The figure shows three views and two pictorial views of one solid part (mm, origin at its lowest corner). Answer the questions. A direction names the side the tool comes from. Round coordinates to 2 decimals unless told otherwise and drop trailing zeros. Order: outer loops, then holes, each group sorted by start corner. A loop starts at its lowest first (then second) coordinate and runs counter-clockwise, first axis right, second up. Notation, with made-up numbers: M -18,30.5 L 13,30.5 A13 ccw 13,39.5 Z; hole C -27.5,-35 d9. An arc over 180 degrees is marked long. Return JSON: item names as keys, results as strings.
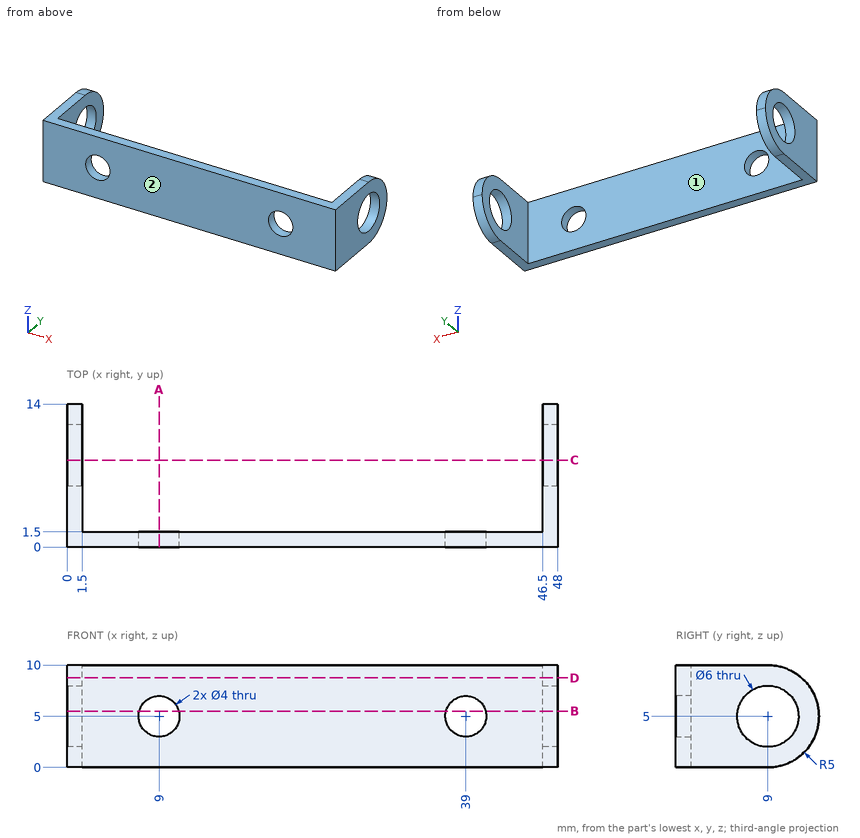
Item 1: Find section C-C (y = 8.5). Determine the outline of the cut face in (x, z).
Output:
{"outline": "M 0,0 L 1.5,0 L 1.5,2.04 L 0,2.04 Z; M 0,7.96 L 1.5,7.96 L 1.5,10 L 0,10 Z; M 46.5,0 L 48,0 L 48,2.04 L 46.5,2.04 Z; M 46.5,7.96 L 48,7.96 L 48,10 L 46.5,10 Z"}
Item 2: This flat-tipped pin is pushed along its axis until it touches: pin 1 (5 mm diameter, centred on x = 20, z = 3, fed in from +Y). Where does it stop, or does it pass through?
Output:
{"pin 1": "stops at y = 1.5"}
Item 3: Consider line 1 along X through (y, z) = (1, 5); line 2 along Y through (x, z) = (47.2, 5); line 3 along X through (y, z) = (3, 9). Determine where each line is inside the solid, lowest interval first. Write a range as [from, to].
Output:
{"line 1": "x = [0, 7], [11, 37], [41, 48]", "line 2": "y = [0, 6], [12, 14]", "line 3": "x = [0, 1.5], [46.5, 48]"}
Item 4: Which of the six approach directions +Z, -Z, +X, -X, +Y, -Y give full straight-line access (tool end or side, diameter ignored) to the marked faces 1 and 2?
Output:
{"face 1": "+Z, -Z, +Y", "face 2": "+Z, -Z, +X, -X, -Y"}
Item 5: Find section D-D (z = 8.75). Determine the outline of the cut face in (x, y), plus the area to 3 significant figures.
Output:
{"outline": "M 0,0 L 48,0 L 48,12.31 L 46.5,12.31 L 46.5,1.5 L 1.5,1.5 L 1.5,12.31 L 0,12.31 Z", "area": "104 mm^2"}
Item 6: Find section B-B (z = 5.5). Determine the outline of the cut face in (x, y), plus the area to 3 significant figures.
Output:
{"outline": "M 0,0 L 7.06,0 L 7.06,1.5 L 1.5,1.5 L 1.5,6.04 L 0,6.04 Z; M 0,11.96 L 1.5,11.96 L 1.5,13.97 L 0,13.97 Z; M 10.94,0 L 37.06,0 L 37.06,1.5 L 10.94,1.5 Z; M 40.94,0 L 48,0 L 48,6.04 L 46.5,6.04 L 46.5,1.5 L 40.94,1.5 Z; M 46.5,11.96 L 48,11.96 L 48,13.97 L 46.5,13.97 Z", "area": "80.1 mm^2"}
Item 7: Find section A-A (x = 9). Determine the outline of the cut face in (y, z).
Output:
{"outline": "M 0,0 L 1.5,0 L 1.5,3 L 0,3 Z; M 0,7 L 1.5,7 L 1.5,10 L 0,10 Z"}
